Source: CAD feature listing. Evaluate the final solid. Frame: model axes, mm. Face numbers are marked on the shaded views. A direction names the side the tool comes from. Give positions to 0.01 mm unless a question says otherwise; leave off trailing zeros. Order: outer loops, then holes, each group sorted by start corner. A loop starts at its lowest first (then second) coordinate and runs counter-clockwise, first axis right, second up.
1) Access query for the marked faces 1 and 2. Directions: +Z, -Z, +X, -X, +Y, -Y. A direction counts if a zero-diameter tool reaches every point of the face in a straight line with its end or side. Return the directions, or none.
2) First-contact query: P1, Ø16.5, axis at x = 23.5, y = -5.5, coming from the +Z side; P2, Ø1.2, axis at x = 3, y = -49.5, coming from the +Z side; P3, Ø7.5, axis at x = -17.5, y = 3, coming from the +Z side. Flat tips, straight axial feed; report the tip coordinate or a pass-through.
3) Section B-B, the plane y = -17.5. Return loops of the section in (x, z).
4) Section C-C, the plane x = 24. Return loops of the section in (y, z), plus the area to 3 significant figures.
5) Section A-A, the plane x = -7.5. Return loops of the section in (y, z), plus the area to 3 significant figures.
6) Section D-D, the plane y = -46.5. Return loops of the section in (x, z).
7) Material intervals for line 1 (Y direction, x = 24, z = 6.35); line 2 (Y direction, x = -24, z = 5.95); line 3 (X direction, y = 17.5, z = 6), sorted ascending.
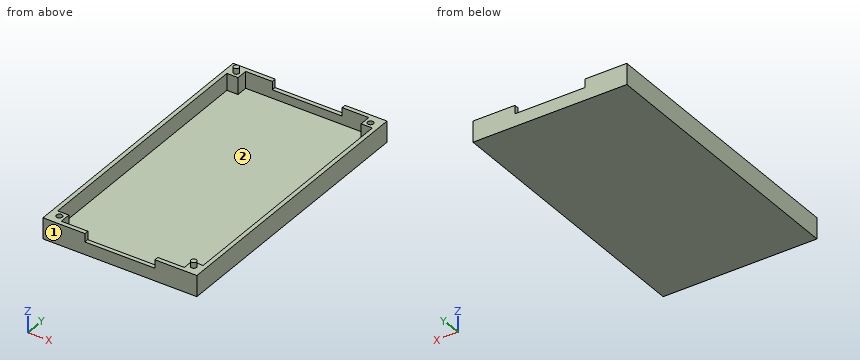
```python
from build123d import *

# Parameters (mm, degrees)
SKETCH_W        = 55
SKETCH_H        = 100
PAD_DEPTH       = 1.5
SKETCH001_W     = 55
SKETCH001_H     = 100
SKETCH001_W_2   = 52
SKETCH001_H_2   = 97
PAD001_DEPTH    = 6
SKETCH002_W     = 25
SKETCH002_H     = 1.5
POCKET_DEPTH    = 3
SKETCH003_W     = 4
SKETCH003_H     = 4
PAD002_DEPTH    = 6
SKETCH004_R     = 1
PAD003_DEPTH    = 2
SKETCH005_R     = 1
PAD004_DEPTH    = 2
SKETCH006_R     = 1.05
POCKET001_DEPTH = 2.5
SKETCH007_R     = 1.05
POCKET002_DEPTH = 2.5


with BuildPart() as part:
    # Sketch → Pad (new body)
    with BuildSketch(Plane.XY):
        Rectangle(SKETCH_W, SKETCH_H)
    extrude(amount=PAD_DEPTH)

    # Sketch001 (on Face6 of Pad) → Pad001 (join)
    with BuildSketch(Plane.XY.offset(1.5)):
        Rectangle(SKETCH001_W, SKETCH001_H)
        Rectangle(SKETCH001_W_2, SKETCH001_H_2, mode=Mode.SUBTRACT)
    extrude(amount=PAD001_DEPTH)

    # Sketch002 (on Face9 of Pad001) → Pocket (cut)
    with BuildSketch(Plane.XY.offset(7.5)):
        with Locations((0, 49.25)):
            Rectangle(SKETCH002_W, SKETCH002_H)
        with Locations((0, -49.25)):
            Rectangle(SKETCH002_W, SKETCH002_H)
    extrude(amount=-POCKET_DEPTH, mode=Mode.SUBTRACT)

    # Sketch003 (on Face22 of Pocket) → Pad002 (join)
    with BuildSketch(Plane.XY.offset(1.5)):
        with Locations((-24, -46.5)):
            Rectangle(SKETCH003_W, SKETCH003_H)
        with Locations((24, -46.5)):
            Rectangle(SKETCH003_W, SKETCH003_H)
        with Locations((24, 46.5)):
            Rectangle(SKETCH003_W, SKETCH003_H)
        with Locations((-24, 46.5)):
            Rectangle(SKETCH003_W, SKETCH003_H)
    extrude(amount=PAD002_DEPTH)

    # Sketch004 (on Face21 of Pad002) → Pad003 (join)
    with BuildSketch(Plane.XY.offset(7.5)):
        with Locations((-24, 46.5)):
            Circle(SKETCH004_R)
    extrude(amount=PAD003_DEPTH)

    # Sketch005 (on Face16 of Pad003) → Pad004 (join)
    with BuildSketch(Plane.XY.offset(7.5)):
        with Locations((24, -46.5)):
            Circle(SKETCH005_R)
    extrude(amount=PAD004_DEPTH)

    # Sketch006 (on Face18 of Pad004) → Pocket001 (cut)
    with BuildSketch(Plane.XY.offset(7.5)):
        with Locations((24, 46.5)):
            Circle(SKETCH006_R)
    extrude(amount=-POCKET001_DEPTH, mode=Mode.SUBTRACT)

    # Sketch007 (on Face22 of Pocket001) → Pocket002 (cut)
    with BuildSketch(Plane.XY.offset(7.5)):
        with Locations((-24, -46.5)):
            Circle(SKETCH007_R)
    extrude(amount=-POCKET002_DEPTH, mode=Mode.SUBTRACT)


solid = part.part
```
From the geometry:
1. face 1: +Z, -Z, +X, -X, -Y
1. face 2: +Z
2. P1: stops at z = 7.5
2. P2: stops at z = 4.5
2. P3: stops at z = 1.5
3. outline: (-27.5, 0) - (27.5, 0) - (27.5, 7.5) - (26, 7.5) - (26, 1.5) - (-26, 1.5) - (-26, 7.5) - (-27.5, 7.5) - close
4. outline: (-50, 0) - (50, 0) - (50, 7.5) - (47.55, 7.5) - (47.55, 5) - (45.45, 5) - (45.45, 7.5) - (44.5, 7.5) - (44.5, 1.5) - (-44.5, 1.5) - (-44.5, 7.5) - (-45.5, 7.5) - (-45.5, 9.5) - (-47.5, 9.5) - (-47.5, 7.5) - (-50, 7.5) - close
4. area: 215 mm2
5. outline: (-50, 0) - (50, 0) - (50, 4.5) - (48.5, 4.5) - (48.5, 1.5) - (-48.5, 1.5) - (-48.5, 4.5) - (-50, 4.5) - close
5. area: 159 mm2
6. outline: (-27.5, 0) - (27.5, 0) - (27.5, 7.5) - (25, 7.5) - (25, 9.5) - (23, 9.5) - (23, 7.5) - (22, 7.5) - (22, 1.5) - (-22, 1.5) - (-22, 7.5) - (-22.95, 7.5) - (-22.95, 5) - (-25.05, 5) - (-25.05, 7.5) - (-27.5, 7.5) - close
7. line 1: y = -50 to -44.5, 44.5 to 45.45, 47.55 to 50
7. line 2: y = -50 to -47.55, -45.45 to -44.5, 44.5 to 50
7. line 3: x = -27.5 to -26, 26 to 27.5
